Answer from the drawing. Dimensions are ordinates in mm from the lowest x, y and z of the part. A direction names the side the tool comes from. Give positions to 0.01 mm unless a question says otherwise; leave off trailing zeros. Loops run counter-clockwise (first coordinate to the right, second up) from the corner with the lowest first, then second, coordinate; pieces in that order, holes last. Notation, with made-up numbers: (-11, 40.5) - (12, 40.5) arc R16 cw to (12, 65.5) - close; hole circle Ø10 at (-13.5, 72). An arc over 180 degrees is marked (long way). Answer as CSV lines item,"result". Start each with the question number.
1) A cutting plane is placed at C-C (z = 91). Determine the outline of the cut face in (x, y).
2) Flat-ended cylindrical pins translate along their axes: pin 1 (3 mm diameter, centred on x = 37.5, y = 41.5, fed in from -Z); pin 2 (4 mm diameter, centred on x = 32.5, z = 85, fed in from -Y); pin 3 (10 mm diameter, centred on y = 37, z = 85.5, fed in from -X). Find the tip coordinate at first contact, or state that the pin passes through.
3) Find the intervals of material crossed by line 1 along Z through (x, y) = (32, 25); line 2 along X through (y, z) = (24, 41); line 3 along X through (y, z) = (13.5, 22.5), in increasing order.
4) For the marked faces 1, 2 and 3, determine the directions among +Z, -Z, +X, -X, +Y, -Y from which every point of the face is accessible in a straight line to the end or side of a thin tool.
5) A cutting plane is placed at D-D (z = 43.5). Determine the outline of the cut face in (x, y), and give its area (3 significant figures).
6) A cutting plane is placed at A-A (x = 24.5). Determine the outline of the cut face in (y, z), and give its area (3 significant figures).
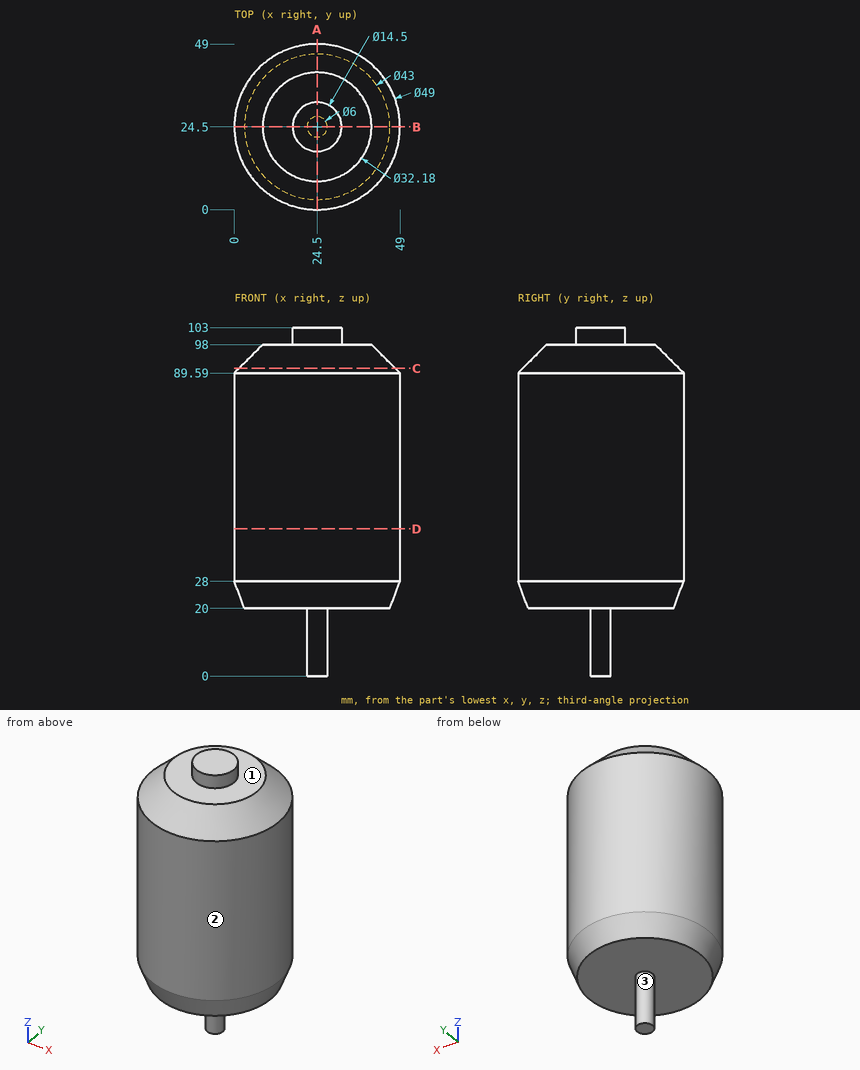
Ans:
1,outline,"circle Ø46.18 at (24.5, 24.5)"
2,pin 1,"z = 20"
2,pin 2,"y = 0.75"
2,pin 3,"x = 1.18"
3,line 1,"20 to 98"
3,line 2,"0.01 to 48.99"
3,line 3,"4.94 to 44.06"
4,face 1,"+Z"
4,face 2,"+Z, -Z"
4,face 3,"-Z"
5,outline,"circle Ø49 at (24.5, 24.5)"
5,area,"1,890 mm2"
6,outline,"(0, 28) - (3, 20) - (21.5, 20) - (21.5, 0) - (27.5, 0) - (27.5, 20) - (46, 20) - (49, 28) - (49, 89.59) - (40.59, 98) - (31.75, 98) - (31.75, 103) - (17.25, 103) - (17.25, 98) - (8.41, 98) - (0, 89.59) - close"
6,area,"3,920 mm2"
